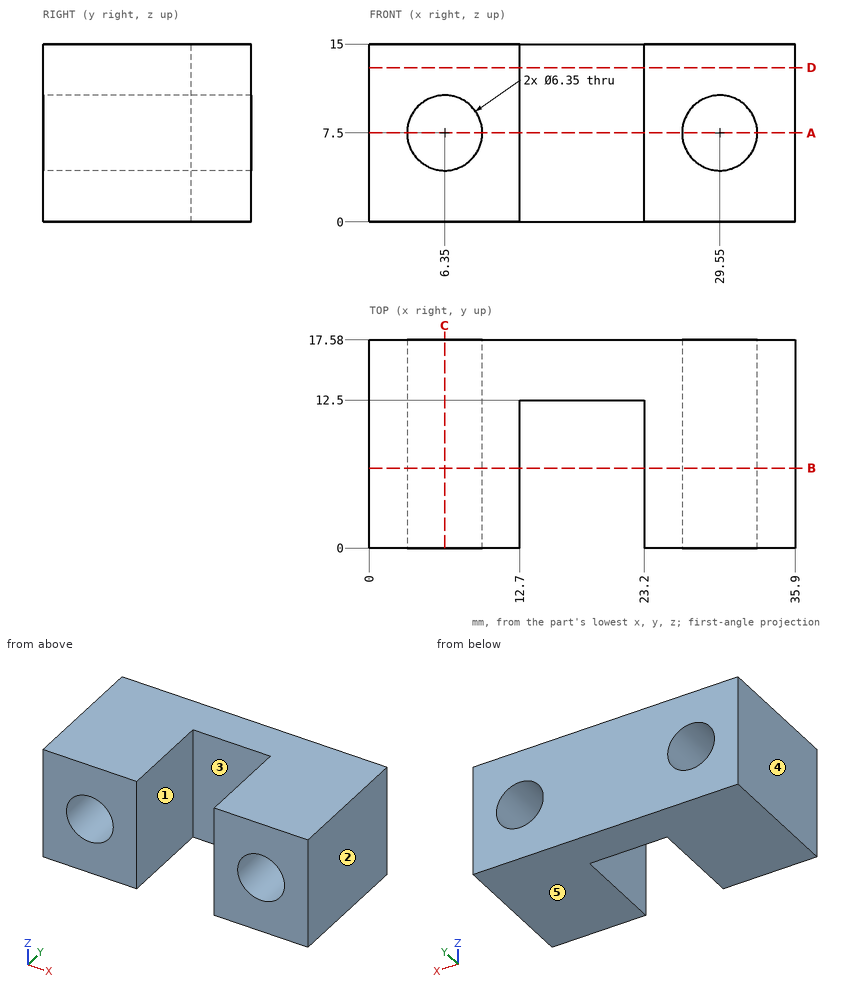
Verification items for this drawing (mm, ordinates from the low corner). A direction names the side the tool comes from. Give positions to 0.01 mm unless a question says otherwise; leave off trailing zeros. Write each loop counter-clockwise with the first axis right and the second up, starting at its lowest first coordinate (ties: lowest second). Pieces come first, ordered by that corner, then holes. Notation, with made-up numbers: (54, 26.25) - (73, 26.25) arc R14 ccw to (73, 49.25) - close; hole circle Ø5 at (34.5, -19.75). An arc over 180 degrees is marked (long way). Answer as a JSON object with one key per item and string values. Group by question number.
1) Thickness scan on probe 1 along Z at (x, y) = (29.55, 8.5) (3 decimals); probe 2 along X at (y, z) = (10.5, 12.75); probe 3 along X at (y, z) = (9.75, 6.75). Record the ranges inside material, lowest first. Write a range as from..to.
2) Sectioned sample at C-C (x = 6.35). Record the cut outline in (y, z) (3 decimals), then the cut area to 3 significant figures.
3) Sectioned sample at D-D (z = 13). Record the cut outline in (x, y), then the cut area to 3 significant figures.
4) Sectioned sample at B-B (y = 6.75). Record the cut outline in (x, z) (3 decimals).
5) Access from +Z, -Z, +X, -X, +Y, -Y to the whole of each face (thin tool, end or side, straight path). Record for the marked faces 1 and 2.
6) Sectioned sample at A-A (z = 7.5). Record the cut outline in (x, y) (3 decimals), then the cut area to 3 significant figures.
7) Release check for a two-part mould opening along X. For the marked faces 3, 4 and 5 record: pulls with the +X half, pulls with the -X half, needs draft (parallel to the pull), parting line crosses it, or undercut.
8) Depth check by flat-ended pin: P1, Ø4, axis at x = 6.35, z = 7.5, coming from the +Y side; P2, Ø5, axis at x = 17.5, z = 10, coming from the -Y side. Enter the tip coordinate at first touch or a pass-through.
Geometry results:
{
 "1": {"probe 1": "z = 0..4.325, 10.675..15", "probe 2": "x = 0..12.7, 23.2..35.9", "probe 3": "x = 0..3.26, 9.44..12.7, 23.2..26.46, 32.64..35.9"},
 "2": {"outline": "(0, 0) - (17.58, 0) - (17.58, 4.325) - (0, 4.325) - close; (0, 10.675) - (17.58, 10.675) - (17.58, 15) - (0, 15) - close", "area": "152 mm^2"},
 "3": {"outline": "(0, 0) - (12.7, 0) - (12.7, 12.5) - (23.2, 12.5) - (23.2, 0) - (35.9, 0) - (35.9, 17.58) - (0, 17.58) - close", "area": "500 mm^2"},
 "4": {"outline": "(0, 0) - (12.7, 0) - (12.7, 15) - (0, 15) - close; (23.2, 0) - (35.9, 0) - (35.9, 15) - (23.2, 15) - close; hole circle Ø6.35 at (6.35, 7.5); hole circle Ø6.35 at (29.55, 7.5)"},
 "5": {"face 1": "+Z, -Z, -Y", "face 2": "+Z, -Z, +X, +Y, -Y"},
 "6": {"outline": "(0, 0) - (3.175, 0) - (3.175, 17.58) - (0, 17.58) - close; (9.525, 0) - (12.7, 0) - (12.7, 12.5) - (23.2, 12.5) - (23.2, 0) - (26.375, 0) - (26.375, 17.58) - (9.525, 17.58) - close; (32.725, 0) - (35.9, 0) - (35.9, 17.58) - (32.725, 17.58) - close", "area": "277 mm^2"},
 "7": {"face 3": "undercut", "face 4": "pulls with the -X half", "face 5": "needs draft"},
 "8": {"P1": "passes through", "P2": "stops at y = 12.5"}
}
